Autodesk Inventor part; units mm, degrees
ref_plane "YZ Plane" through (0, 0, 0) normal (1, 0, 0) x (0, 1, 0)
ref_plane "XZ Plane" through (0, 0, 0) normal (0, 1, 0) x (-1, 0, 0)
ref_plane "XY Plane" through (0, 0, 0) normal (0, 0, 1) x (1, 0, 0)
sketch "Sketch1" plane through (0, 0, 0) normal (0, 0, 1) x (1, 0, 0)
  line L0 (0, 0) -> (-101.6, 0)
  line L1 (-101.6, 0) -> (-101.6, 12.7)
  line L2 (-101.6, 12.7) -> (-12.7, 12.7)
  line L3 (0, 12.7) -> (0, 0)
  line L4 (0, 0) -> (-12.7, 0)
  line L5 (-12.7, 12.7) -> (-12.7, 76.2)
  line L6 (-12.7, 76.2) -> (88.9, 76.2)
  line L7 (88.9, 76.2) -> (88.9, 63.5)
  line L8 (88.9, 63.5) -> (0, 63.5)
  line L9 (0, 63.5) -> (0, 12.7)
  dimension "d0" = 101.6
  dimension "d4" = 12.7
  dimension "d5" = 12.7
  dimension "d6" = 12.7
  dimension "d7" = 76.2
  dimension "d8" = 101.6
  dimension "d9" = 12.7
  dimension "d10" = 88.9
extrude "Extrusion1" add sketch "Sketch1" along normal mid plane 25.4
fillet "Fillet1" radius 12.7 1 edges at (88.9, 69.85, -12.7)
fillet "Fillet2" radius 12.7 1 edges at (88.9, 69.85, 12.7)
fillet "Fillet3" radius 12.7 1 edges at (-101.6, 6.35, -12.7)
fillet "Fillet4" radius 12.7 1 edges at (-101.6, 6.35, 12.7)
sketch "Sketch2" plane through (-12.7, 12.7, 12.7) normal (0, 1, 0) x (1, 0, 0)
  arc A0 (-76.2, 25.4) -> (-76.2, 0) centre (-76.2, 12.7) ccw
  circle A1 centre (-76.2, 12.7) radius 6.35
  point P0 (12.7, 12.7)
  dimension "d17" = 12.7
extrude "Extrusion2" cut sketch "Sketch2" against normal blind 25.4
sketch "Sketch3" plane through (-12.7, 76.2, 12.7) normal (0, 1, 0) x (1, 0, 0)
  arc A0 (88.9, 0) -> (88.9, 25.4) centre (88.9, 12.7) ccw
  point P0 (12.7, 12.7)
hole "Hole1" at (76.2, 76.2, 0) direction (0, -1, 0) diameter 6.35 end through all counterbore diameter 12.7 counterbore depth 1.5875
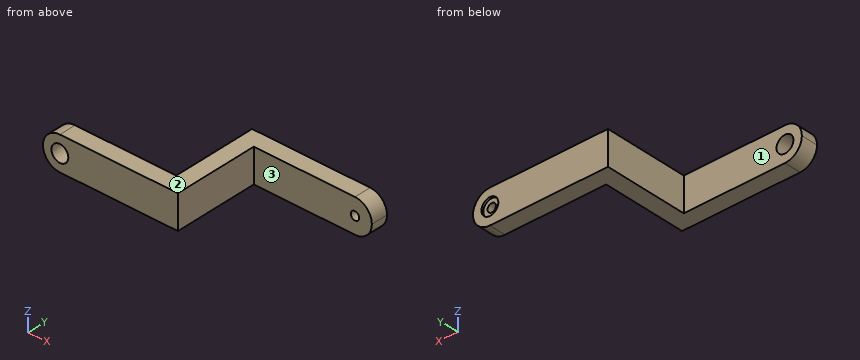
Could you check a few things on this model? Use its own coordinates, in mm. Face numbers are marked on the shaded views. A direction names the side the tool comes from. Give positions to 0.01 mm unless a question says otherwise; leave off trailing zeros. Order: outer loops, then holes, each group sorted by start corner. A loop starts at its lowest first (then second) coordinate and runs counter-clockwise, first axis right, second up. Notation, with made-up numbers: (70, 10.5) - (125, 10.5) arc R17 cw to (125, 15.5) - close; hole circle Ø3 at (47, -36.5). An arc over 180 degrees is marked (long way). One line per item, written item: value. Start each with the question number.
1. For P1, Ø12.5, axis at x = 66.5, z = 5, coming from the -Y side; P2, Ø8, axis at y = 30.5, z = -3.5, coming from the +X side; P3, Ø14.5, axis at x = -88.9, z = 0, coming from the +Y side, each with a flat end and sliding along its axis, tell me the tip position at first contact or that it passes through.
2. For the marked faces 1, 2 and 3, which set-ups out of +Z, -Z, +X, -X, +Y, -Y let a thin tool reach every point of the face, with its end or its side?
3. If I drill on probe 1 along Z at (x, y) = (76.2, 65.75) (3 decimals); probe 2 along Z at (x, y) = (76.2, 75.25); probe 3 along X at (y, z) = (5, 0), over which ranges is the centre line in solid material (lowest first)?
4. Imagine slicing it at B-B on y = 56. List the corners of the cut face in (x, z) for me.
5. Imagine slicing it at C-C on x = -37. List the corners of the cut face in (y, z) for me.
Values:
1. P1: y = 63.5
1. P2: x = 0
1. P3: y = 12.7
2. face 1: +Z, -Z, -X, +Y
2. face 2: +Z, +X, -X, +Y, -Y
2. face 3: +Z, -Z, +X, -Y
3. probe 1: -12.7 to -3.175, 3.175 to 12.7
3. probe 2: -12.7 to -6.35, 6.35 to 12.7
3. probe 3: -101.6 to -95.25, -82.55 to 0
4. outline: (-12.7, -12.7) - (0, -12.7) - (0, 12.7) - (-12.7, 12.7) - close
5. outline: (0, -12.7) - (12.7, -12.7) - (12.7, 12.7) - (0, 12.7) - close
